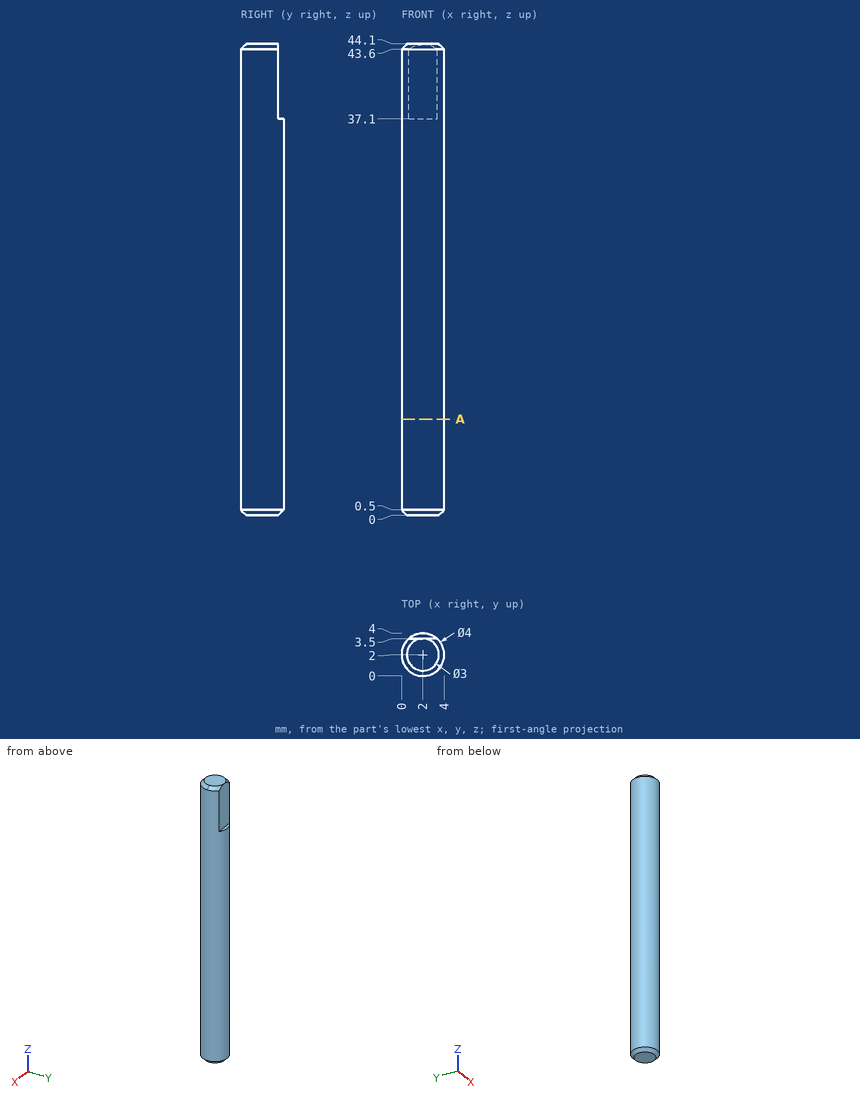
Verification items for this drawing (mm, ordinates from the low corner). Round coordinates to 2 decimals unless told otherwise and drop trailing zeros. Write each loop counter-clockwise with the first axis right and the second up, starting at its lowest first coordinate (ties: lowest second). Pieces come first, ordered by that corner, then holes. Notation, with made-up numbers: (-31.5, 24) - (-26.5, 24) arc R22 cw to (-26.5, 52) - close; hole circle Ø11 at (51, 60.25). An arc over 180 degrees is marked (long way). Answer as a JSON object with one key per item and string values. Group by question number.
Q1. Section check A-A, the plane z = 9. Enter the section's corners in (x, y).
Q2. Go/stop test with flat-tipped pins: pin 1 Ø1 at (y, z) = (3, 8) entering from +X; pin 2 Ø0.8 at (x, z) = (2, 41.5) entering from +Y. Record where each tip stops, or that it passes through.
Q3. Thickness scan on line 1 (X direction, y = 3.35, z = 11) (1 decimal); line 2 (X direction, y = 2.8, z = 30); line 3 (Y direction, x = 2.9, z = 6). Record the ranges inside material, lowest first.
Found:
{
 "1": {"outline": "circle Ø4 at (2, 2)"},
 "2": {"pin 1": "stops at x = 3.94", "pin 2": "stops at y = 3.5"},
 "3": {"line 1": "x = 0.5 to 3.5", "line 2": "x = 0.17 to 3.83", "line 3": "y = 0.21 to 3.79"}
}
